```python
from build123d import *

# Parameters (mm, degrees)
SKETCH_1_R               = 12.5
EXTRUDE_1_DEPTH          = 16
SKETCH_2_R               = 16
EXTRUDE_2_DEPTH          = 10
SKETCH_3_R               = 28
EXTRUDE_3_DEPTH          = 6
SKETCH_6_R               = 2
CUT_EXTRUDE_1_DEPTH      = 10
PATTERN_CIRCULAR_2_COUNT = 4
SKETCH_8_R               = 16
EXTRUDE_5_DEPTH          = 10
SKETCH_7_R               = 7.5
EXTRUDE_6_DEPTH          = 80


with BuildPart() as part:
    # 草图1 → 凸台-拉伸1 (new body)
    with BuildSketch(Plane.XY):
        Circle(SKETCH_1_R)
    extrude(amount=EXTRUDE_1_DEPTH)

    # 草图2 → 凸台-拉伸2 (add)
    with BuildSketch(Plane.XY.offset(16)):
        Circle(SKETCH_2_R)
    extrude(amount=EXTRUDE_2_DEPTH)

    # 草图3 → 凸台-拉伸3 (add)
    with BuildSketch(Plane.XY.offset(26)):
        Circle(SKETCH_3_R)
    extrude(amount=EXTRUDE_3_DEPTH)

    # 草图6 → 切除-拉伸1 (cut)
    with BuildSketch(Plane(origin=(0, 0, 26), x_dir=(-1, 0, 0), z_dir=(0, 0, -1))):
        with Locations((0, 21)):
            Circle(SKETCH_6_R)
    cut_extrude_1 = extrude(amount=-CUT_EXTRUDE_1_DEPTH, mode=Mode.SUBTRACT)

    # 阵列(圆周)2: 切除-拉伸1 ×4 about axis
    pattern_circular_2_axis = Axis((0, 0, 0), (0, 0, 1))
    for i in range(1, PATTERN_CIRCULAR_2_COUNT):
        add(cut_extrude_1.rotate(pattern_circular_2_axis, i * 360 / PATTERN_CIRCULAR_2_COUNT), mode=Mode.SUBTRACT)

    # 草图8 → 凸台-拉伸5 (add)
    with BuildSketch(Plane.XY.offset(32)):
        Circle(SKETCH_8_R)
    extrude(amount=EXTRUDE_5_DEPTH)

    # 草图7 → 凸台-拉伸6 (add)
    with BuildSketch(Plane(origin=(0, 0, 0), x_dir=(-1, 0, 0), z_dir=(0, 0, -1))):
        Circle(SKETCH_7_R)
    extrude(amount=EXTRUDE_6_DEPTH)


solid = part.part
```
Check sheet for the modelled part. Datum: model origin and axes. Units: mm. A direction names the side the tool comes from. Coordinates: 2 decimals unless noted, no trailing zeros. Order: outer loops, then holes, each group sorted by start corner. A loop starts at its lowest first (then second) coordinate and runs counter-clockwise, first axis right, second up. Notation, with made-up numbers: (30, 46.25) -> (66, 46.25) arc R28 cw to (66, 84.25) -> close; hole circle Ø8 at (1.5, 61). An arc over 180 degrees is marked (long way). Write item = value, one per line. Start each with the question number.
1) Material ranges on L1, parallel to Y at x = 0, z = 28.6; L2, parallel to Z at x = 7, y = -4; L3, parallel to X at y = 0.5, z = -17.5, recorded low to high.
2) Go/stop test with flat-tipped pins: P1, Ø5, axis at x = 0, y = -21, coming from the +Z side; P2, Ø12, axis at x = 3.5, z = -17, coming from the -Y side; P3, Ø5, axis at y = 6.5, z = 12, coming from the -X side. Record where each tip stops, or that it passes through.
3) Mould release check, pull along X, two halves, no side actions. Record for faces 4 (the flat face through (0, 0, 42)), 5 (the cylindrical face through (0, -23, 29)), 6 (the cylindrical face through (-3.47, -15.62, 20.93)), 7 (the cylindrical face through (23, 0, 29)): +X half, -X half, draft (parallel to the pull), parting line (faces both ways), or undercut.
4) Cross-section at A-A (y = 0). Enter the section's corners in (x, z).
5) Access from +Z, -Z, +X, -X, +Y, -Y to the whole of each face (thin tool, end or side, straight path). Record for faces 1 (the cylindrical face through (25.865, -10.724, 28.958)), 2 (the cylindrical face through (7.493, 0.33, -39.44)), 3 (the cylindrical face through (-3.47, -15.62, 36.93)).
6) Cross-section at C-C (y = 21). Enter the section's corners in (x, z), then the cut area to 3 significant figures.
Ans:
q1.L1 = -28 to -23, -19 to 19, 23 to 28
q1.L2 = 0 to 42
q1.L3 = -7.48 to 7.48
q2.P1 = 32
q2.P2 = -7.5
q2.P3 = -11.84
q3.face_4 = draft
q3.face_5 = undercut
q3.face_6 = parting line
q3.face_7 = undercut
q4.outline = (-28, 26) -> (-23, 26) -> (-23, 32) -> (-28, 32) -> close; (-19, 26) -> (-16, 26) -> (-16, 16) -> (-12.5, 16) -> (-12.5, 0) -> (-7.5, 0) -> (-7.5, -80) -> (7.5, -80) -> (7.5, 0) -> (12.5, 0) -> (12.5, 16) -> (16, 16) -> (16, 26) -> (19, 26) -> (19, 32) -> (16, 32) -> (16, 42) -> (-16, 42) -> (-16, 32) -> (-19, 32) -> close; (23, 26) -> (28, 26) -> (28, 32) -> (23, 32) -> close
q5.face_1 = +Z, -Z
q5.face_2 = -Z
q5.face_3 = +Z
q6.outline = (-18.52, 26) -> (-2, 26) -> (-2, 32) -> (-18.52, 32) -> close; (2, 26) -> (18.52, 26) -> (18.52, 32) -> (2, 32) -> close
q6.area = 198 mm²
